```python
from build123d import *

# Parameters (mm, degrees)
SKETCH_2_R          = 4
SKETCH_2_R_2        = 2
EXTRUDE_1_DEPTH     = 56
CUT_EXTRUDE_1_REACH = 27
SKETCH_3_W          = 52
SKETCH_3_H          = 64
CUT_EXTRUDE_2_REACH = 4
SKETCH_4_R          = 4
SKETCH_4_R_2        = 2
FILLET_1_R          = 2
FILLET_2_R          = 2


with BuildPart() as part:
    # 草图2 → 凸台-拉伸1 (new body)
    with BuildSketch(Plane(origin=(0, 0, 0), x_dir=(0, 0, -1), z_dir=(1, 0, 0))):
        with BuildLine():
            Line((-23.249580799, 25.750000985), (-23.249580799, -25.75))
            Line((-23.249580799, -25.75), (1.750419201, -25.75))
            Line((1.750419201, -25.75), (1.750419201, 25.75))
            ThreePointArc((1.750419201, 25.75), (-10.749580306, 38.250000985), (-23.249580799, 25.750000985))
        make_face()
        with Locations((-10.749580799, 25.750000985)):
            Circle(SKETCH_2_R, mode=Mode.SUBTRACT)
        with Locations((-10.749580799, 32.750000985)):
            Circle(SKETCH_2_R_2, mode=Mode.SUBTRACT)
        with Locations((-17.749579814, 25.75000197)):
            Circle(SKETCH_2_R_2, mode=Mode.SUBTRACT)
        with Locations((-10.749580799, 18.750002956)):
            Circle(SKETCH_2_R_2, mode=Mode.SUBTRACT)
        with Locations((-3.749581784, 25.75000197)):
            Circle(SKETCH_2_R_2, mode=Mode.SUBTRACT)
    extrude(amount=EXTRUDE_1_DEPTH)

    # 草图3 → 切除-拉伸1 (cut, up to next)
    with BuildSketch(Plane(origin=(0, 0, -1.750419201), x_dir=(-1, 0, 0), z_dir=(0, 0, -1)), mode=Mode.PRIVATE) as cut_extrude_1_sk1:
        with Locations((-28, 8.25)):
            Rectangle(SKETCH_3_W, SKETCH_3_H)
    cut_extrude_1_tool1 = extrude(cut_extrude_1_sk1.sketch, amount=-CUT_EXTRUDE_1_REACH, mode=Mode.PRIVATE) & part.part
    add(cut_extrude_1_tool1.solids().sort_by_distance((28, 8.25, -1.750419))[0], mode=Mode.SUBTRACT)

    # 草图4 → 切除-拉伸2 (cut, up to next)
    with BuildSketch(Plane(origin=(0, -23.75, 0), x_dir=(1, 0, 0), z_dir=(0, 1, 0)), mode=Mode.PRIVATE) as cut_extrude_2_sk1:
        with Locations((28, -10.749580799)):
            Circle(SKETCH_4_R)
    cut_extrude_2_tool1 = extrude(cut_extrude_2_sk1.sketch, amount=-CUT_EXTRUDE_2_REACH, mode=Mode.PRIVATE) & part.part
    add(cut_extrude_2_tool1.solids().sort_by_distance((28, -23.75, 10.749581))[0], mode=Mode.SUBTRACT)
    # 草图4 → 切除-拉伸2 (cut, up to next)
    with BuildSketch(Plane(origin=(0, -23.75, 0), x_dir=(1, 0, 0), z_dir=(0, 1, 0)), mode=Mode.PRIVATE) as cut_extrude_2_sk2:
        with Locations((35, -10.749580799)):
            Circle(SKETCH_4_R_2)
    cut_extrude_2_tool2 = extrude(cut_extrude_2_sk2.sketch, amount=-CUT_EXTRUDE_2_REACH, mode=Mode.PRIVATE) & part.part
    add(cut_extrude_2_tool2.solids().sort_by_distance((35, -23.75, 10.749581))[0], mode=Mode.SUBTRACT)
    # 草图4 → 切除-拉伸2 (cut, up to next)
    with BuildSketch(Plane(origin=(0, -23.75, 0), x_dir=(1, 0, 0), z_dir=(0, 1, 0)), mode=Mode.PRIVATE) as cut_extrude_2_sk3:
        with Locations((28, -17.749580799)):
            Circle(SKETCH_4_R_2)
    cut_extrude_2_tool3 = extrude(cut_extrude_2_sk3.sketch, amount=-CUT_EXTRUDE_2_REACH, mode=Mode.PRIVATE) & part.part
    add(cut_extrude_2_tool3.solids().sort_by_distance((28, -23.75, 17.749581))[0], mode=Mode.SUBTRACT)
    # 草图4 → 切除-拉伸2 (cut, up to next)
    with BuildSketch(Plane(origin=(0, -23.75, 0), x_dir=(1, 0, 0), z_dir=(0, 1, 0)), mode=Mode.PRIVATE) as cut_extrude_2_sk4:
        with Locations((21, -10.749580799)):
            Circle(SKETCH_4_R_2)
    cut_extrude_2_tool4 = extrude(cut_extrude_2_sk4.sketch, amount=-CUT_EXTRUDE_2_REACH, mode=Mode.PRIVATE) & part.part
    add(cut_extrude_2_tool4.solids().sort_by_distance((21, -23.75, 10.749581))[0], mode=Mode.SUBTRACT)
    # 草图4 → 切除-拉伸2 (cut, up to next)
    with BuildSketch(Plane(origin=(0, -23.75, 0), x_dir=(1, 0, 0), z_dir=(0, 1, 0)), mode=Mode.PRIVATE) as cut_extrude_2_sk5:
        with Locations((28, -3.749580799)):
            Circle(SKETCH_4_R_2)
    cut_extrude_2_tool5 = extrude(cut_extrude_2_sk5.sketch, amount=-CUT_EXTRUDE_2_REACH, mode=Mode.PRIVATE) & part.part
    add(cut_extrude_2_tool5.solids().sort_by_distance((28, -23.75, 3.749581))[0], mode=Mode.SUBTRACT)
    # 草图4 → 切除-拉伸2 (cut, up to next)
    with BuildSketch(Plane(origin=(0, -23.75, 0), x_dir=(1, 0, 0), z_dir=(0, 1, 0)), mode=Mode.PRIVATE) as cut_extrude_2_sk6:
        with Locations((8, -10.749580799)):
            Circle(SKETCH_4_R_2)
    cut_extrude_2_tool6 = extrude(cut_extrude_2_sk6.sketch, amount=-CUT_EXTRUDE_2_REACH, mode=Mode.PRIVATE) & part.part
    add(cut_extrude_2_tool6.solids().sort_by_distance((8, -23.75, 10.749581))[0], mode=Mode.SUBTRACT)
    # 草图4 → 切除-拉伸2 (cut, up to next)
    with BuildSketch(Plane(origin=(0, -23.75, 0), x_dir=(1, 0, 0), z_dir=(0, 1, 0)), mode=Mode.PRIVATE) as cut_extrude_2_sk7:
        with Locations((48, -10.749580799)):
            Circle(SKETCH_4_R_2)
    cut_extrude_2_tool7 = extrude(cut_extrude_2_sk7.sketch, amount=-CUT_EXTRUDE_2_REACH, mode=Mode.PRIVATE) & part.part
    add(cut_extrude_2_tool7.solids().sort_by_distance((48, -23.75, 10.749581))[0], mode=Mode.SUBTRACT)

    # 圆角1
    fillet_1_edges = [part.edges().sort_by_distance(p)[0] for p in [
        (56, -25.75, 10.749580799),
    ]]
    fillet(fillet_1_edges, radius=FILLET_1_R)

    # 圆角2
    fillet_2_edges = [part.edges().sort_by_distance(p)[0] for p in [
        (0, -25.75, 10.749580799),
    ]]
    fillet(fillet_2_edges, radius=FILLET_2_R)


solid = part.part
```
For this review, take the finished solid that the model builds, in its own axes (mm). A direction names the side the tool comes from. Round coordinates to 2 decimals unless told otherwise and drop trailing zeros. Write each loop counter-clockwise with the first axis right and the second up, starting at its lowest first coordinate (ties: lowest second). Pieces come first, ordered by that corner, then holes.
1) Insertion check: pin 1 Ø3 at (y, z) = (25.75, 17.75) entering from -X; pin 2 Ø13 at (y, z) = (25.75, 10.75) entering from -X; pin 3 Ø2 at (x, z) = (33, 11) entering from +Y. Each pin has a flat end and moves straight along its axis. Give the tip position at first contact, or say it passes through.
Answer below:
pin 1: passes through
pin 2: stops at x = 0
pin 3: stops at y = -23.75
2) Machinability: for faces 1 (the face through (2, 7, 11)), 2 (the face through (54.986, 27.733, 18.01)), which of the approach directions +Z, -Z, +X, -X, +Y, -Y give a long, thin tool a straight path to every point of the face, cutting with its end or side? Answer none if there is none.
Answer below:
face 1: +Z, -Z, +Y
face 2: +X, -X
3) Take a section at A-A on x = 28. Give the boundary of the cut face in (y, z), then the cut area to 3 significant figures.
Answer below:
outline: (-25.75, -1.75) - (-23.75, -1.75) - (-23.75, 1.75) - (-25.75, 1.75) - close; (-25.75, 5.75) - (-23.75, 5.75) - (-23.75, 6.75) - (-25.75, 6.75) - close; (-25.75, 14.75) - (-23.75, 14.75) - (-23.75, 15.75) - (-25.75, 15.75) - close; (-25.75, 19.75) - (-23.75, 19.75) - (-23.75, 23.25) - (-25.75, 23.25) - close
area: 18.0 mm2
4) For line 1 along Z through (x, y) = (28, -25); line 2 along X through (y, z) = (-12, 2); line 3 along Y through (x, z) = (49, 14.5), list the stretches that pass through material, from the lowest coordinate up.
Answer below:
line 1: z = -1.75 to 1.75, 5.75 to 6.75, 14.75 to 15.75, 19.75 to 23.25
line 2: x = 0 to 2, 54 to 56
line 3: y = -25.75 to -23.75
5) Take a section at D-D on y = 32.75. Give the boundary of the cut face in (x, z).
Answer below:
outline: (0, 0.39) - (2, 0.39) - (2, 8.75) - (0, 8.75) - close; (0, 12.75) - (2, 12.75) - (2, 21.11) - (0, 21.11) - close; (54, 0.39) - (56, 0.39) - (56, 8.75) - (54, 8.75) - close; (54, 12.75) - (56, 12.75) - (56, 21.11) - (54, 21.11) - close
6) Take a section at C-C on y = 3. Give the boundary of the cut face in (x, z).
Answer below:
outline: (0, -1.75) - (2, -1.75) - (2, 23.25) - (0, 23.25) - close; (54, -1.75) - (56, -1.75) - (56, 23.25) - (54, 23.25) - close
7) Mouldability with a two-part tool opening along Y and no side actions: class faces 3 (the face through (22, -25.75, 8)), 4 (the face through (54.986, 20.102, 12.224)), 5 (the face through (24.826, -24.736, 13.184)), 6 (the face through (54.986, 38.247, 10.475)) as +Y half, -Y half, draft (parallel to the pull), parting line (faces both ways), or undercut.
Answer below:
face 3: -Y half
face 4: undercut
face 5: draft
face 6: +Y half
8) Take a section at B-B on x = 8. Give the boundary of the cut face in (y, z), then the cut area to 3 significant figures.
Answer below:
outline: (-25.75, -1.75) - (-23.75, -1.75) - (-23.75, 8.75) - (-25.75, 8.75) - close; (-25.75, 12.75) - (-23.75, 12.75) - (-23.75, 23.25) - (-25.75, 23.25) - close
area: 42.0 mm2
